Verification items for the finished model (mm, model axes). A direction names the side the tool comes from. Coordinates: 2 decimals unless noted, no trailing zeros. Write each loop counter-clockwise with the first axis right and the second up, starting at its lowest first coordinate (ties: lowest second). Pieces come first, ordered by that corner, then holes. Notation, with made-up numbers: (-9, 60.25) -> (4, 60.25) arc R22 cw to (4, 86.25) -> close; hole circle Ø9 at (72.5, 72). An arc over 180 degrees is marked (long way). Answer in a Markdown table with one row per item.
```python
from build123d import *

# Parameters (mm, degrees)
SKETCH1_W                        = 36.4
SKETCH1_H                        = 9.8
BOSS_EXTRUDE1_DEPTH              = 4
SKETCH2_W                        = 4
SKETCH2_H                        = 6.999999999
CUT_EXTRUDE1_DEPTH               = 5
SKETCH3_W                        = 4
SKETCH3_H                        = 6.999999999
CUT_EXTRUDE2_DEPTH               = 5
F_2_05_2_05_DIAMETER_HOLE1_D     = 2.05
F_2_05_2_05_DIAMETER_HOLE1_DEPTH = 6.35
F_2_05_2_05_DIAMETER_HOLE1_TIP   = 0.615882135
F_2_05_2_05_DIAMETER_HOLE2_D     = 2.05
F_2_05_2_05_DIAMETER_HOLE2_DEPTH = 9.8
CHAMFER1_SIZE                    = 1


with BuildPart() as part:
    # Sketch1 → Boss-Extrude1 (new body)
    with BuildSketch(Plane(origin=(0, 4, 0), x_dir=(1, 0, 0), z_dir=(0, 1, 0))):
        with Locations((0, -4.9)):
            Rectangle(SKETCH1_W, SKETCH1_H)
    extrude(amount=-BOSS_EXTRUDE1_DEPTH)

    # Sketch2 → Cut-Extrude1 (cut, through all)
    with BuildSketch(Plane.XZ):
        with Locations((-16.2, 3.5)):
            Rectangle(SKETCH2_W, SKETCH2_H)
    extrude(amount=-CUT_EXTRUDE1_DEPTH, mode=Mode.SUBTRACT)

    # Sketch3 → Cut-Extrude2 (cut, through all)
    with BuildSketch(Plane.XZ):
        with Locations((16.2, 3.5)):
            Rectangle(SKETCH3_W, SKETCH3_H)
    extrude(amount=-CUT_EXTRUDE2_DEPTH, mode=Mode.SUBTRACT)

    # Ø2.05 (2.05) Diameter Hole1
    with Locations(Plane(origin=(0, 0, 0), x_dir=(-1, 0, 0), z_dir=(0, 0, -1))):
        with Locations((10, 2), (-10, 2)):
            Hole(F_2_05_2_05_DIAMETER_HOLE1_D / 2, depth=F_2_05_2_05_DIAMETER_HOLE1_DEPTH)
            with Locations((0, 0, -(F_2_05_2_05_DIAMETER_HOLE1_DEPTH + F_2_05_2_05_DIAMETER_HOLE1_TIP / 2))):  # 118° drill point
                Cone(0, F_2_05_2_05_DIAMETER_HOLE1_D / 2, F_2_05_2_05_DIAMETER_HOLE1_TIP, mode=Mode.SUBTRACT)

    # Ø2.05 (2.05) Diameter Hole2
    with Locations(Plane.XY.offset(9.8)):
        with Locations((16.2, 2)):
            Hole(F_2_05_2_05_DIAMETER_HOLE2_D / 2, depth=F_2_05_2_05_DIAMETER_HOLE2_DEPTH)

    # Chamfer1
    chamfer1_edges = [part.edges().sort_by_distance(p)[0] for p in [
        (-14.2, 2, 0),
        (14.2, 2, 0),
    ]]
    chamfer(chamfer1_edges, length=CHAMFER1_SIZE)


solid = part.part
```
1. Section check A-A, the plane x = 16.2. Record the boundary of the cut face in (y, z) (3 decimals).
Geometry says:
| item | result |
|---|---|
| outline | (0, 7) -> (0.975, 7) -> (0.975, 9.8) -> (0, 9.8) -> close; (3.025, 7) -> (4, 7) -> (4, 9.8) -> (3.025, 9.8) -> close |
2. Tool access check on faces 1 (the cylindrical face through (8.976, 2.045, 3.219)), 2 (the flat face through (18.2, 2, 8)), 3 (the flat face through (15, 2, 7)), 4 (the flat face through (-16, 2, 7)). Record the directions out of +Z, -Z, +X, -X, +Y, -Y that give a thin tool (end or side, any length) a straight path to the whole face; none if there is none.
Geometry says:
| item | result |
|---|---|
| face 1 | -Z |
| face 2 | +Z, -Z, +X, +Y, -Y |
| face 3 | -Z, +X, +Y, -Y |
| face 4 | -Z, -X, +Y, -Y |
3. Thickness scan on line 1 (X direction, y = 2.1, z = 4.5); line 2 (Y direction, x = -10, z = 3) (3 decimals); line 3 (X direction, y = 1.4, z = 1.5). Record the ranges inside material, lowest first. Write a range as from..to.
Geometry says:
| item | result |
|---|---|
| line 1 | -14.2..-11.02, -8.98..8.98, 11.02..14.2 |
| line 2 | 0..0.975, 3.025..4 |
| line 3 | -14.2..-10.83, -9.17..9.17, 10.83..14.2 |
4. Depth check by flat-ended pin: P1, Ø1.8, axis at x = 16.2, y = 2, coming from the -Z side; P2, Ø1.5, axis at x = -6, z = 1.5, coming from the -Y side; P3, Ø1.2, axis at y = 2.5, z = 5, coming from the -X side. Enter the tip coordinate at first touch or a pass-through.
Geometry says:
| item | result |
|---|---|
| P1 | through |
| P2 | y = 0 |
| P3 | x = -14.2 |
5. Section check C-C, the plane y = 3.4. Record the boundary of the cut face in (x, z), plus the area to 3 significant figures.
Geometry says:
| item | result |
|---|---|
| outline | (-18.2, 7) -> (-14.2, 7) -> (-14.2, 1) -> (-13.2, 0) -> (13.2, 0) -> (14.2, 1) -> (14.2, 7) -> (18.2, 7) -> (18.2, 9.8) -> (-18.2, 9.8) -> close |
| area | 300 mm^2 |
6. Section check B-B, the plane z = 7.5. Record the boundary of the cut face in (x, y) (3 decimals).
Geometry says:
| item | result |
|---|---|
| outline | (-18.2, 0) -> (18.2, 0) -> (18.2, 4) -> (-18.2, 4) -> close; hole circle Ø2.05 at (16.2, 2) |
7. Mould release check, pull along X, two halves, no side actions. Record for faces 5 (the flat face through (0, 0, 5)), 6 (the flat face through (-14.2, 2, 4)), 7 (the cylindrical face through (17.224, 2.045, 8.38)): released by +X, released by -X, zero draft, split by the parting line, or undercut.
Geometry says:
| item | result |
|---|---|
| face 5 | zero draft |
| face 6 | released by -X |
| face 7 | undercut |
8. Section check D-D, the plane z = 4.5. Record the boundary of the cut face in (x, y) (3 decimals).
Geometry says:
| item | result |
|---|---|
| outline | (-14.2, 0) -> (14.2, 0) -> (14.2, 4) -> (-14.2, 4) -> close; hole circle Ø2.05 at (-10, 2); hole circle Ø2.05 at (10, 2) |
